from build123d import *

# Parameters (mm, degrees)
SKETCH1_R           = 2
BOSS_EXTRUDE1_DEPTH = 30
SKETCH2_W           = 24
SKETCH2_H           = 18
CUT_EXTRUDE1_DEPTH  = 48.136701039
FILLET1_R           = 5
FILLET2_R           = 2


with BuildPart() as part:
    # Sketch1 → Boss-Extrude1 (new body)
    with BuildSketch(Plane.XY):
        with BuildLine():
            Line((-10, -13.032253728), (-10, 26.967746272))
            ThreePointArc((-10, 26.967746272), (0, 30.36228886), (10, 26.967746272))
            Line((10, 26.967746272), (10, -13.032253728))
            ThreePointArc((10, -13.032253728), (0, -16.426796317), (-10, -13.032253728))
        make_face()
        with Locations((0, -7.032253728)):
            Circle(SKETCH1_R, mode=Mode.SUBTRACT)
        with Locations((6, -7.032253728)):
            Circle(SKETCH1_R, mode=Mode.SUBTRACT)
        with Locations((-6, -7.032253728)):
            Circle(SKETCH1_R, mode=Mode.SUBTRACT)
        with Locations(Location((6, 20.967746272, 0), (0, 0, 180))):
            Circle(SKETCH1_R, mode=Mode.SUBTRACT)
        with Locations(Location((0, 20.967746272, 0), (0, 0, 180))):
            Circle(SKETCH1_R, mode=Mode.SUBTRACT)
        with Locations(Location((-6, 20.967746272, 0), (0, 0, 180))):
            Circle(SKETCH1_R, mode=Mode.SUBTRACT)
    extrude(amount=BOSS_EXTRUDE1_DEPTH)

    # Sketch2 → Cut-Extrude1 (cut, through all)
    with BuildSketch(Plane(origin=(10, 0, 0), x_dir=(0, 0, -1), z_dir=(1, 0, 0))):
        with Locations((-15, -7.426796317)):
            Rectangle(SKETCH2_W, SKETCH2_H)
        with Locations((-15, 21.36228886)):
            Rectangle(SKETCH2_W, SKETCH2_H)
    extrude(amount=-CUT_EXTRUDE1_DEPTH, mode=Mode.SUBTRACT)

    # Fillet1
    fillet1_edges = [part.edges().sort_by_distance(p)[0] for p in [
        (0, 1.573203683, 3),
        (0, 1.573203683, 27),
        (0, 12.36228886, 27),
        (0, 12.36228886, 3),
    ]]
    fillet(fillet1_edges, radius=FILLET1_R)

    # Fillet2
    fillet2_edges = [part.edges().sort_by_distance(p)[0] for p in [
        (0, -16.426796317, 30),
        (10, 6.967746272, 30),
        (0, 30.36228886, 30),
        (10, 6.967746272, 0),
        (0, -16.426796317, 0),
        (-10, 6.967746272, 0),
        (0, 30.36228886, 0),
        (-10, 6.967746272, 30),
    ]]
    fillet(fillet2_edges, radius=FILLET2_R - 0.0001)  # a hair under: the kernel refuses the full size


solid = part.part
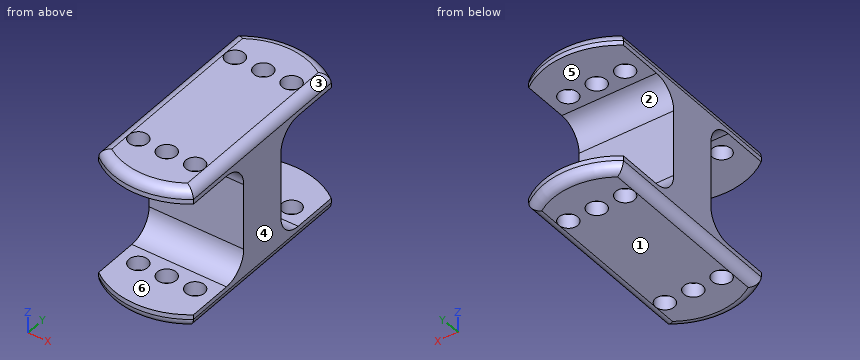
Verification items for the finished model (mm, model axes). Face numbers are marked on the shaded views. A direction names the side the tool comes from. Round coordinates to 2 decimals unless told otherwise and drop trailing zeros. Write each loop counter-clockwise with the first axis right and the second up, starting at its lowest first coordinate (ties: lowest second). Pieces come first, ordered by that corner, then holes.
(1) Material ranges on line 1 (Y direction, x = 0, z = 1.85); line 2 (Y direction, x = -6, z = 27.8); line 3 (Z direction, x = -4.75, y = -9), recorded low to high.
Returned:
line 1: y = -16.42 to -9.03, -5.03 to 18.97, 22.97 to 30.36
line 2: y = -15.29 to -9.03, -5.03 to 18.97, 22.97 to 29.23
line 3: z = 0 to 3, 27 to 30
(2) Section check A-A (y = 0). Enter the section's corners in (x, z), plus the area to 3 significant figures.
Returned:
outline: (-10, 2) arc R2 ccw to (-8, 0) - (8, 0) arc R2 ccw to (10, 2) - (10, 4.36) - (-10, 4.36) - close; (-10, 25.64) - (10, 25.64) - (10, 28) arc R2 ccw to (8, 30) - (-8, 30) arc R2 ccw to (-10, 28) - close
area: 171 mm2
(3) Depth check by flat-ended pin: pin 1 Ø2.5 at (x, y) = (-6, -7.03) entering from +Z; pin 2 Ø6.5 at (x, y) = (0, -7.03) entering from -Z; pin 3 Ø2 at (x, z) = (7.5, 8) entering from +Y; pin 4 Ø10 at (x, z) = (5.5, 5) entering from +Y. Enter the tip coordinate at first touch or a pass-through.
Returned:
pin 1: passes through
pin 2: stops at z = 0
pin 3: stops at y = 12.46
pin 4: stops at y = 30.34
(4) Mould release check, pull along Z, two halves, no side actions. Record for the marked faces 1, 2 and 3: pulls with the +Z half, pulls with the -Z half, needs draft (parallel to the pull), parting line crosses it, or undercut.
Returned:
face 1: pulls with the -Z half
face 2: undercut
face 3: pulls with the +Z half
(5) Section check B-B (x = 0). Give the number of separate pieces and of enclosed holes in the cut face, plus the area to 3 significant figures.
Returned:
separate pieces: 5
enclosed holes: 0
area: 510 mm2
(6) Access from +Z, -Z, +X, -X, +Y, -Y to the whole of each face (thin tool, end or side, straight path). Record for the marked faces 4, 5 and 6.
Returned:
face 4: +Z, -Z, +X, +Y, -Y
face 5: +X, -X, +Y
face 6: +X, -X, -Y
(7) Section check C-C (z = 5.5). Enter the section's corners in (x, y), plus the area to 3 significant figures.
Returned:
outline: (-10, 0.9) - (10, 0.9) - (10, 13.03) - (-10, 13.03) - close
area: 243 mm2
